```python
from build123d import *

# Parameters (mm, degrees)
SKETCH1_W          = 35.56
SKETCH1_H          = 41.148
EXTRUDE1_DEPTH     = 3.175
SKETCH2_W          = 3.175
SKETCH2_H          = 18.923
SKETCH2_H_2        = 15.875
CUT_EXTRUDE3_DEPTH = 4.175
SKETCH3_W          = 29.21
SKETCH3_H          = 6.35
CUT_EXTRUDE4_DEPTH = 4.175
SKETCH4_W          = 3.81
SKETCH4_H          = 3.81
CUT_EXTRUDE5_DEPTH = 4.175


with BuildPart() as part:
    # Sketch1 → Extrude1 (new body)
    with BuildSketch(Plane(origin=(0, 0, 0), x_dir=(0, 0, -1), z_dir=(1, 0, 0))):
        with Locations((17.78, 20.574)):
            Rectangle(SKETCH1_W, SKETCH1_H)
    extrude(amount=EXTRUDE1_DEPTH)

    # Sketch2 → Cut-Extrude3 (cut, through all)
    with BuildSketch(Plane(origin=(3.175, 0, 0), x_dir=(0, 0, -1), z_dir=(1, 0, 0))):
        with Locations((1.5875, 31.6865)):
            Rectangle(SKETCH2_W, SKETCH2_H)
        with Locations((33.9725, 31.6865)):
            Rectangle(SKETCH2_W, SKETCH2_H)
        with Locations((33.9725, 7.9375)):
            Rectangle(SKETCH2_W, SKETCH2_H_2)
        with Locations((1.5875, 7.9375)):
            Rectangle(SKETCH2_W, SKETCH2_H_2)
    extrude(amount=-CUT_EXTRUDE3_DEPTH, mode=Mode.SUBTRACT)

    # Sketch3 → Cut-Extrude4 (cut, through all)
    with BuildSketch(Plane(origin=(3.175, 0, 0), x_dir=(0, 0, -1), z_dir=(1, 0, 0))):
        with Locations((17.78, 3.175)):
            Rectangle(SKETCH3_W, SKETCH3_H)
    extrude(amount=-CUT_EXTRUDE4_DEPTH, mode=Mode.SUBTRACT)

    # Sketch4 → Cut-Extrude5 (cut, through all)
    with BuildSketch(Plane(origin=(3.175, 0, 0), x_dir=(0, 0, -1), z_dir=(1, 0, 0))):
        with Locations((14.485579349, 9.525)):
            Rectangle(SKETCH4_W, SKETCH4_H)
        with Locations((7.896738046, 9.525)):
            Rectangle(SKETCH4_W, SKETCH4_H)
        with Locations((21.074420651, 9.525)):
            Rectangle(SKETCH4_W, SKETCH4_H)
        with Locations((27.663261954, 9.525)):
            Rectangle(SKETCH4_W, SKETCH4_H)
        with Locations((14.485579349, 15.113)):
            Rectangle(SKETCH4_W, SKETCH4_H)
        with Locations((7.896738046, 15.113)):
            Rectangle(SKETCH4_W, SKETCH4_H)
        with Locations((21.074420651, 15.113)):
            Rectangle(SKETCH4_W, SKETCH4_H)
        with Locations((27.663261954, 15.113)):
            Rectangle(SKETCH4_W, SKETCH4_H)
        with Locations((14.485579349, 20.701)):
            Rectangle(SKETCH4_W, SKETCH4_H)
        with Locations((7.896738046, 20.701)):
            Rectangle(SKETCH4_W, SKETCH4_H)
        with Locations((21.074420651, 20.701)):
            Rectangle(SKETCH4_W, SKETCH4_H)
        with Locations((27.663261954, 20.701)):
            Rectangle(SKETCH4_W, SKETCH4_H)
        with Locations((14.485579349, 26.289)):
            Rectangle(SKETCH4_W, SKETCH4_H)
        with Locations((7.896738046, 26.289)):
            Rectangle(SKETCH4_W, SKETCH4_H)
        with Locations((21.074420651, 26.289)):
            Rectangle(SKETCH4_W, SKETCH4_H)
        with Locations((27.663261954, 26.289)):
            Rectangle(SKETCH4_W, SKETCH4_H)
        with Locations((14.485579349, 31.877)):
            Rectangle(SKETCH4_W, SKETCH4_H)
        with Locations((7.896738046, 31.877)):
            Rectangle(SKETCH4_W, SKETCH4_H)
        with Locations((21.074420651, 31.877)):
            Rectangle(SKETCH4_W, SKETCH4_H)
        with Locations((27.663261954, 31.877)):
            Rectangle(SKETCH4_W, SKETCH4_H)
        with Locations((14.485579349, 37.465)):
            Rectangle(SKETCH4_W, SKETCH4_H)
        with Locations((7.896738046, 37.465)):
            Rectangle(SKETCH4_W, SKETCH4_H)
        with Locations((21.074420651, 37.465)):
            Rectangle(SKETCH4_W, SKETCH4_H)
        with Locations((27.663261954, 37.465)):
            Rectangle(SKETCH4_W, SKETCH4_H)
    extrude(amount=-CUT_EXTRUDE5_DEPTH, mode=Mode.SUBTRACT)


solid = part.part
```
The listing builds one solid part. Answer for the finished solid, in the listing's coordinates (mm). A direction names the side the tool comes from. Give positions to 0.01 mm unless a question says otherwise; leave off trailing zeros. Order: outer loops, then holes, each group sorted by start corner. A loop starts at its lowest first (then second) coordinate and runs counter-clockwise, first axis right, second up. Notation, with made-up numbers: (21.25, 83) -> (71.25, 83) arc R10 cw to (71.25, 100) -> close; hole circle Ø6 at (74, 49.25). An arc over 180 degrees is marked (long way). Write each question's results on one line, items separated by ' | '.
Q1. Each of these flat-tipped pins is pushed along its axis until it touches: P1, Ø1.6, axis at x = 2.5, y = 37, coming from the -Z side (3 decimals); P2, Ø1.6, axis at x = 2, y = 10, coming from the +Z side (3 decimals). Where does it stop, or does it pass through?
Checked values:
P1: stops at z = -32.385 | P2: stops at z = -3.175
Q2. Straight lines are drawn through the part: probe 1 along Z at (x, y) = (1.35, 19); probe 2 along Z at (x, y) = (1.1, 31) (3 decimals); probe 3 along Z at (x, y) = (1.35, 24) (3 decimals). For each, find the intervals that lie inside material, in ascending order. Write a range as from..to.
Checked values:
probe 1: z = -35.56..-29.57, -25.76..-22.98, -19.17..-16.39, -12.58..-9.8, -5.99..0 | probe 2: z = -32.385..-29.568, -25.758..-22.979, -19.169..-16.391, -12.581..-9.802, -5.992..-3.175 | probe 3: z = -32.385..-3.175
Q3. The part is cut by section A-A, the plane y = 20.5. Give the vertices of the cut face in (x, z) (3 decimals).
Checked values:
outline: (0, -35.56) -> (3.175, -35.56) -> (3.175, -29.568) -> (0, -29.568) -> close; (0, -25.758) -> (3.175, -25.758) -> (3.175, -22.979) -> (0, -22.979) -> close; (0, -19.169) -> (3.175, -19.169) -> (3.175, -16.391) -> (0, -16.391) -> close; (0, -12.581) -> (3.175, -12.581) -> (3.175, -9.802) -> (0, -9.802) -> close; (0, -5.992) -> (3.175, -5.992) -> (3.175, 0) -> (0, 0) -> close
Q4. The part is cut by section D-D, the plane x = 0.65. State how many separate pieces and enclosed holes the cut face has, and give its area (3 significant figures).
Checked values:
separate pieces: 1 | enclosed holes: 24 | area: 708 mm^2
Q5. The part is cut by section C-C, the plane y = 38. Give the vertices of the cut face in (x, z) (3 decimals).
Checked values:
outline: (0, -32.385) -> (3.175, -32.385) -> (3.175, -29.568) -> (0, -29.568) -> close; (0, -25.758) -> (3.175, -25.758) -> (3.175, -22.979) -> (0, -22.979) -> close; (0, -19.169) -> (3.175, -19.169) -> (3.175, -16.391) -> (0, -16.391) -> close; (0, -12.581) -> (3.175, -12.581) -> (3.175, -9.802) -> (0, -9.802) -> close; (0, -5.992) -> (3.175, -5.992) -> (3.175, -3.175) -> (0, -3.175) -> close
Q6. The part is cut by section B-B, the plane z = -20. Give the vertices of the cut face in (x, y) (3 decimals).
Checked values:
outline: (0, 6.35) -> (3.175, 6.35) -> (3.175, 7.62) -> (0, 7.62) -> close; (0, 11.43) -> (3.175, 11.43) -> (3.175, 13.208) -> (0, 13.208) -> close; (0, 17.018) -> (3.175, 17.018) -> (3.175, 18.796) -> (0, 18.796) -> close; (0, 22.606) -> (3.175, 22.606) -> (3.175, 24.384) -> (0, 24.384) -> close; (0, 28.194) -> (3.175, 28.194) -> (3.175, 29.972) -> (0, 29.972) -> close; (0, 33.782) -> (3.175, 33.782) -> (3.175, 35.56) -> (0, 35.56) -> close; (0, 39.37) -> (3.175, 39.37) -> (3.175, 41.148) -> (0, 41.148) -> close
Q7. Determine the mould class of faces 3 (the face through (2, 11, -3.175)), 4 (the face through (2, 22.606, -8)) for opening direction Y: pulls with the +Y half, pulls with the -Y half, needs draft (parallel to the pull), parting line crosses it, or undercut.
Checked values:
face 3: needs draft | face 4: undercut
Q8. Which of the six approach directions +Z, -Z, +X, -X, +Y, -Y give full straight-line access (tool end or side, diameter ignored) to faces 1 (the face through (2, 39.37, -8)), 2 (the face through (2, 32, -32.385))?
Checked values:
face 1: +X, -X | face 2: -Z, +X, -X, +Y
